Autodesk Inventor part; units mm, degrees
ref_plane "YZ Plane" through (0, 0, 0) normal (1, 0, 0) x (0, 1, 0)
ref_plane "XZ Plane" through (0, 0, 0) normal (0, 1, 0) x (-1, 0, 0)
ref_plane "XY Plane" through (0, 0, 0) normal (0, 0, 1) x (1, 0, 0)
sketch "Эскиз1" plane through (0, 0, 0) normal (1, 0, 0) x (0, 1, 0)
  circle A0 centre (0, 0) radius 20
  dimension "d0" = 40
extrude "Выдавливание1" add sketch "Эскиз1" along normal blind 19
sketch "Эскиз2" plane through (19, 0, 0) normal (1, 0, 0) x (0, 0, -1)
  circle A0 centre (0, 0) radius 3
  dimension "d3" = 6
extrude "Выдавливание2" add sketch "Эскиз2" along normal blind 2
sketch "Эскиз3" plane through (21, 0, 0) normal (1, 0, 0) x (0, 0, -1)
  circle A0 centre (0, 0) radius 2.25
  dimension "d6" = 4.5
extrude "Выдавливание3" cut sketch "Эскиз3" against normal blind 100
fillet "Сопряжение1" radius 1 2 edges at (0, -20, 0) (19, -20, 0)
fillet "Сопряжение2" radius 2 1 edges at (19, 0, 3)
properties part number "каток"
Geometry: final body of the model. Coordinates: model frame, mm. Give positions to 0.01 mm unless a question says otherwise; leave off trailing zeros. Order: outer loops, then holes, each group sorted by start corner. A loop starts at its lowest first (then second) coordinate and runs counter-clockwise, first axis right, second up. Notation, with made-up numbers: (30.5, -30.75) - (65.5, -30.75) arc R24 ccw to (65.5, -20.75) - close; hole circle Ø2 at (3.25, -26). An arc over 180 degrees is marked (long way). Use CSV: the item, a comma, the result in double quotes.
1. Contact query for flat-ended pins moving along their axis: pin 1 (1 mm diameter, centred on x = 3.5, z = -10.5, fed in from -Y); pin 2 (8 mm diameter, centred on x = 12.5, y = -4.5, fed in from +Z); pin 3 (11.5 mm diameter, centred on y = 8, z = 8, fed in from +X); pin 4 (12 mm diameter, centred on x = 14, z = 6, fed in from -Y). Output: stop coordinate, or through.
Answers below:
pin 1,"y = -17.32"
pin 2,"z = 19.99"
pin 3,"x = 19"
pin 4,"y = -20"
2. Mould query, pull axis Z, two halves, no side actions, for faces 1 (the face through (9.381, -4.336, 19.524)), 2 (the face through (10.65, 2.23, 0.29)), 3 (the face through (0, 0, -4)). Classes: +Z half, -Z half, draft (parallel to the pull), parting line (faces both ways), or undercut.
Answers below:
face 1,"parting line"
face 2,"undercut"
face 3,"draft"
3. Section query C-C (x = 5.75). Output: boundary loops of the cut face in (y, z), plus the area to 3 significant figures.
Answers below:
outline,"circle Ø40 at (0, 0); hole circle Ø4.5 at (0, 0)"
area,"1,240 mm2"
4. Material intervals for line 1 along X through (y, z) = (-12.5, -11.5); line 2 along Z through (x, y) = (7, 3.5); line 3 along Z through (x, y) = (4.5, 6.5), sorted ascending. Write a range as from..to.
Answers below:
line 1,"0..19"
line 2,"-19.69..19.69"
line 3,"-18.91..18.91"
